Verification items for this drawing (mm, ordinates from the low corner). A direction names the side the tool comes from. Round coordinates to 2 decimals unless told otherwise and drop trailing zeros. Order: outer loops, then holes, each group sorted by start corner. A loop starts at its lowest first (then second) coordinate and runs counter-clockwise, first axis right, second up. Notation, with made-up numbers: (76.5, 53) -> (116.5, 53) arc R15 cw to (116.5, 60) -> close; hole circle Ø6 at (51.5, 65). An arc over 180 degrees is marked (long way). Answer in a Markdown table with one row per item.
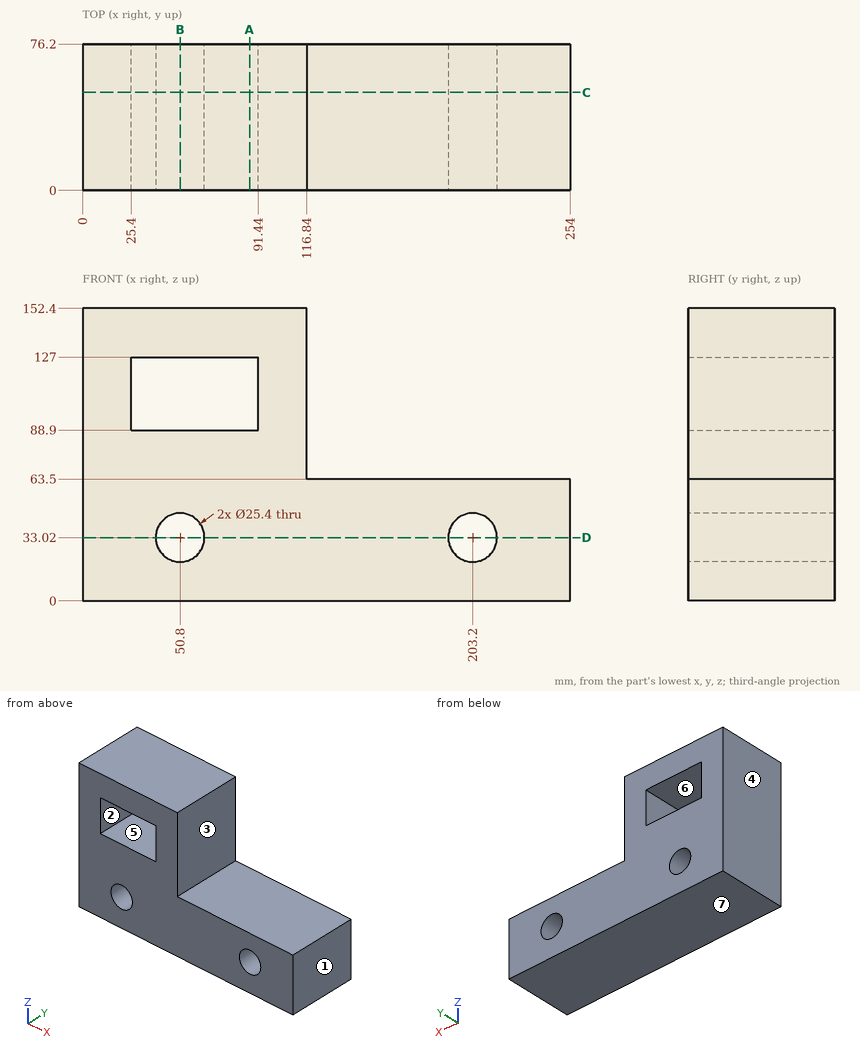
Item 1: Depth check by flat-ended pin: P1, Ø20.5, axis at x = 203.2, z = 33.02, coming from the -Y side; P2, Ø23, axis at x = 187.5, y = 36.5, coming from the +Z side; P3, Ø19, axis at y = 54.5, z = 102, coming from the +X side. Enter the tip coordinate at first touch or a pass-through.
Result sheet:
| item | result |
|---|---|
| P1 | passes through |
| P2 | stops at z = 63.5 |
| P3 | stops at x = 116.84 |
Item 2: Set-up check for the marked faces 1, 2 and 3: record each of +Z, -Z, +X, -X, +Y, -Y from which the full face is reachable in a straight line by a thin tool's end or side.
Result sheet:
| item | result |
|---|---|
| face 1 | +Z, -Z, +X, +Y, -Y |
| face 2 | +Y, -Y |
| face 3 | +Z, +X, +Y, -Y |
Item 3: Cross-section at C-C (y = 51). Record the boundary of the cut face in (x, z), and give its area (3 significant figures).
Result sheet:
| item | result |
|---|---|
| outline | (0, 0) -> (254, 0) -> (254, 63.5) -> (116.84, 63.5) -> (116.84, 152.4) -> (0, 152.4) -> close; hole (25.4, 88.9) -> (91.44, 88.9) -> (91.44, 127) -> (25.4, 127) -> close; hole circle Ø25.4 at (50.8, 33.02); hole circle Ø25.4 at (203.2, 33.02) |
| area | 23,000 mm^2 |
Item 4: Mould release check, pull along X, two halves, no side actions. Record for the marked faces 4, 5, 6 and 7: pulls with the +X half, pulls with the -X half, needs draft (parallel to the pull), parting line crosses it, or undercut.
Result sheet:
| item | result |
|---|---|
| face 4 | pulls with the -X half |
| face 5 | undercut |
| face 6 | undercut |
| face 7 | needs draft |
Item 5: Scan lines: line 1 (Z direction, x = 50.8, y = 54); line 2 (Z direction, x = 90, y = 52); line 3 (Z direction, x = 203.2, y = 61). Record each from-to range of solid material in increasing order. Write a range as [from, to].
Result sheet:
| item | result |
|---|---|
| line 1 | z = [0, 20.32], [45.72, 88.9], [127, 152.4] |
| line 2 | z = [0, 88.9], [127, 152.4] |
| line 3 | z = [0, 20.32], [45.72, 63.5] |
Item 6: Cross-section at B-B (x = 50.8). Record the boundary of the cut face in (y, z).
Result sheet:
| item | result |
|---|---|
| outline | (0, 0) -> (76.2, 0) -> (76.2, 20.32) -> (0, 20.32) -> close; (0, 45.72) -> (76.2, 45.72) -> (76.2, 88.9) -> (0, 88.9) -> close; (0, 127) -> (76.2, 127) -> (76.2, 152.4) -> (0, 152.4) -> close |
Item 7: Cross-section at A-A (x = 87). Record the boundary of the cut face in (y, z), and give its area (3 significant figures).
Result sheet:
| item | result |
|---|---|
| outline | (0, 0) -> (76.2, 0) -> (76.2, 88.9) -> (0, 88.9) -> close; (0, 127) -> (76.2, 127) -> (76.2, 152.4) -> (0, 152.4) -> close |
| area | 8,710 mm^2 |
Item 8: Cross-section at D-D (z = 33.02). Record the boundary of the cut face in (x, y), and give its area (3 significant figures).
Result sheet:
| item | result |
|---|---|
| outline | (0, 0) -> (38.1, 0) -> (38.1, 76.2) -> (0, 76.2) -> close; (63.5, 0) -> (190.5, 0) -> (190.5, 76.2) -> (63.5, 76.2) -> close; (215.9, 0) -> (254, 0) -> (254, 76.2) -> (215.9, 76.2) -> close |
| area | 15,500 mm^2 |
